Input: part model. Units: mm. Frame: model coordinates. A direction names the side the tool comes from. Round coordinates to 2 decimals unless told otherwise and drop trailing zeros. Loops run counter-clockwise (first coordinate to the right, second up) from the corner with the lowest first, then second, coordinate; pieces in that order, holes last. Notation, with made-up numbers: (23.5, 58.5) -> (27.5, 58.5) arc R7 cw to (27.5, 71.5) -> close; hole circle Ø3 at (46, 33). An arc over 180 degrees is marked (long way). Answer as a JSON object with one key per item and string values. Group by question number.
Item 1: Pin query (flat end, axial travel): pin 1 (8 mm diameter, centred on x = -25.5, z = -9, fed in from -Y); pin 2 (1.5 mm diameter, centred on x = 32, y = -25.5, fed in from +Z); pin 3 (1 mm diameter, centred on x = 1.5, z = -11, fed in from +Y). Return the tip coordinate at first contact, or that it passes through.
Item 2: Set-up query: faces 4 (the cylindrical face through (40.1, 0.09, -15.07)), 5 (the cylindrical face through (-3.47, -15.62, -5.56)). Return all of +Z, -Z, +X, -X, +Y, -Y with unobstructed straight access to the full face (end or side cutting, diameter ignored); none if empty.
Item 3: Draft query along Y for faces 1 (the flat face through (9.4, -19.4, -10)), 2 (the cylindrical face through (-14.985, 0.66, -15.07)), 3 (the cylindrical face through (20.765, -39.923, -14.93)). Return one class per face: released by +Y, released by -Y, zero draft, split by the parting line, or undercut.
Item 4: Section query D-D on z = -3.5. Return loops of the section in (x, y), and give its area (3 significant figures).
Item 5: Section query C-C on z = -15.25. Return loops of the section in (x, y).
Item 6: Section query A-A on y = 0. Return loops of the section in (x, z).
Item 7: Section query B-B on x = -38. Return loops of the section in (y, z), and give its area (3 significant figures).
Item 8: Material intervals for line 1 (Y direction, x = 0.5, z = -1.75); line 2 (Y direction, x = 6, z = -12); line 3 (Z direction, x = -15, y = 4.5), sorted ascending. Write a range as [from, to].
from build123d import *

# Parameters (mm, degrees)
CHAMFER1_SIZE     = 1
CHAMFER1_SIZE2    = 0.267949192
M5_TAPPED_HOLE1_D = 4.2


with BuildPart() as part:
    # Sketch1 → Revolve1 (revolve)
    with BuildSketch(Plane(origin=(0, 0, 0), x_dir=(1, 0, 0), z_dir=(0, 1, 0))):
        Polygon((16, 0), (16, 10), (15, 10), (15, 20), (45, 20), (45, 10), (21, 10), (21, 0), align=None)
    revolve(axis=Axis((0, 0, 0), (0, 0, 1)))

    # Chamfer1
    chamfer1_edges = [part.edges().sort_by_distance(p)[0] for p in [
        (-16, 0, 0),
    ]]
    chamfer1_side = [part.faces().sort_by_distance(p)[0] for p in [
        (-16, 0, -5),
    ]]
    chamfer(chamfer1_edges, length=CHAMFER1_SIZE, length2=CHAMFER1_SIZE2, reference=chamfer1_side[0])

    # M5 Tapped Hole1 (through all)
    with Locations(Plane.XY.offset(-10)):
        with Locations((-38, 0), (38, 0)):
            Hole(M5_TAPPED_HOLE1_D / 2)


solid = part.part
Solved:
{
 "1": {"pin 1": "y = -39.46", "pin 2": "z = -10", "pin 3": "y = 44.99"},
 "2": {"face 4": "+Z, -Z", "face 5": "+Z"},
 "3": {"face 1": "zero draft", "face 2": "undercut", "face 3": "split by the parting line"},
 "4": {"outline": "circle Ø42 at (0, 0); hole circle Ø32 at (0, 0)", "area": "581 mm²"},
 "5": {"outline": "circle Ø90 at (0, 0); hole circle Ø4.2 at (-38, 0); hole circle Ø30 at (0, 0); hole circle Ø4.2 at (38, 0)"},
 "6": {"outline": "(-45, -20) -> (-40.1, -20) -> (-40.1, -10) -> (-45, -10) -> close; (-35.9, -20) -> (-15, -20) -> (-15, -10) -> (-16, -10) -> (-16, -1) -> (-16.27, 0) -> (-21, 0) -> (-21, -10) -> (-35.9, -10) -> close; (15, -20) -> (35.9, -20) -> (35.9, -10) -> (21, -10) -> (21, 0) -> (16.27, 0) -> (16, -1) -> (16, -10) -> (15, -10) -> close; (40.1, -20) -> (45, -20) -> (45, -10) -> (40.1, -10) -> close"},
 "7": {"outline": "(-24.1, -20) -> (-2.1, -20) -> (-2.1, -10) -> (-24.1, -10) -> close; (2.1, -20) -> (24.1, -20) -> (24.1, -10) -> (2.1, -10) -> close", "area": "440 mm²"},
 "8": {"line 1": "[-20.99, -15.99], [15.99, 20.99]", "line 2": "[-44.6, -13.75], [13.75, 44.6]", "line 3": "[-20, -10]"}
}
